Could you check a few things on this drawing? It's one solid part, dimensions in mm from its lowest x, y, z. A direction names the side the tool comes from. Give positions to 0.01 mm unless a question says otherwise; leave off trailing zeros. Order: outer loops, then holes, each group sorted by start corner. A loop starts at its lowest first (then second) coordinate and runs counter-clockwise, first axis right, second up.
(1) Imagine slicing it at D-D, the plane z = 2.5. Write out the boundary of the cut face in (x, y), then the cut area to 3 significant figures.
(2) If I drill on probe 1 along X at (y, z) = (46.85, 6); probe 2 along Z at (x, y) = (45, 48.2); probe 3 along Y at (x, z) = (14.5, 3), over which ranges is the centre line in solid material (lowest first)?
(3) On a 3-axis mill with a long thin cutter (end or side, diameter ignored), from which of +Z, -Z, +X, -X, +Y, -Y can I reach the whole of each face in a straight line? I mean the marked faces 5 and 6. Say none if no direction works.
(4) If we mould it in two halves opening along X, with no side actions, what happens to the marked faces 1, 2, 3 and 4? For each: released by +X, released by -X, zero draft, split by the parting line, or undercut.
(5) Imagine slicing it at A-A, the plane x = 25. Write out the boundary of the cut face in (y, z), then the cut area to 3 significant figures.
(6) Imagine slicing it at C-C, the plane x = 45. Write out the boundary of the cut face in (y, z).
(7) Will these pins go through, and if not, where does the flat tip stop? pin 1 (4 mm diameter, centred on x = 4, z = 6, fed in from +Y); pin 2 (1.5 mm diameter, centred on x = 45.5, z = 6.5, fed in from -Y).
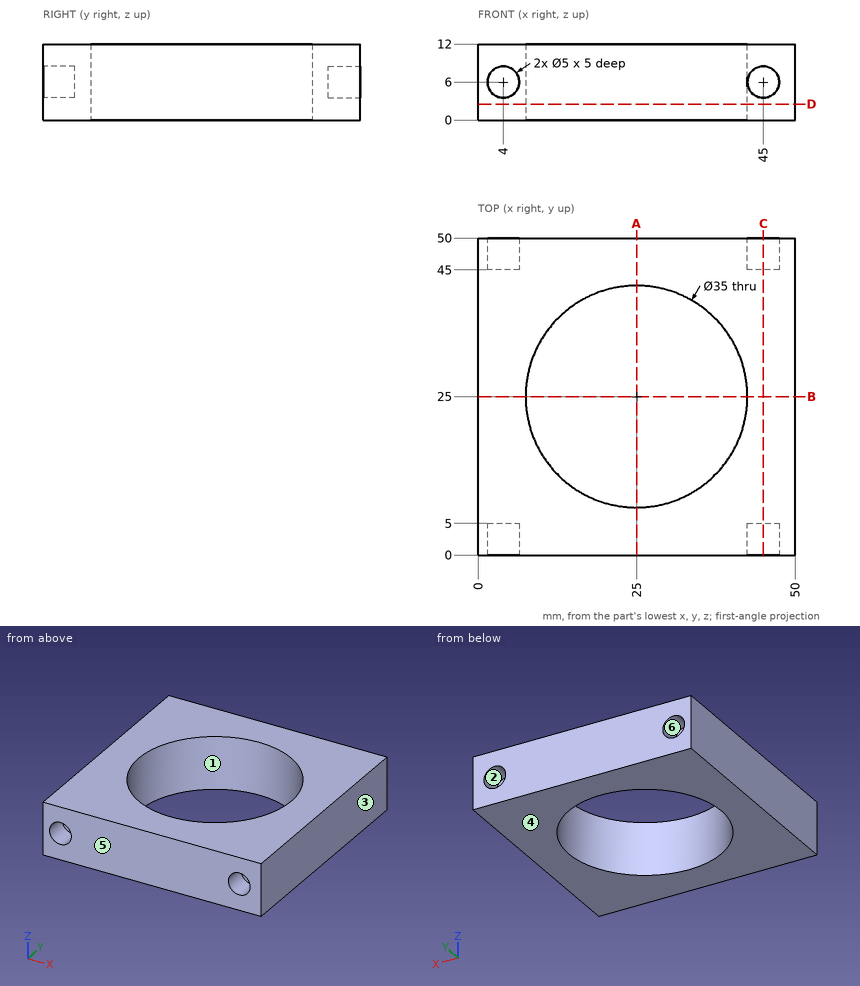
Answer block:
1. outline: (0, 0) - (50, 0) - (50, 50) - (0, 50) - close; hole circle Ø35 at (25, 25)
1. area: 1,540 mm2
2. probe 1: x = 0 to 1.5, 6.5 to 42.5, 47.5 to 50
2. probe 2: z = 0 to 3.5, 8.5 to 12
2. probe 3: y = 0 to 11, 39 to 50
3. face 5: +Z, -Z, +X, -X, -Y
3. face 6: +Y
4. face 1: undercut
4. face 2: undercut
4. face 3: released by +X
4. face 4: zero draft
5. outline: (0, 0) - (7.5, 0) - (7.5, 12) - (0, 12) - close; (42.5, 0) - (50, 0) - (50, 12) - (42.5, 12) - close
5. area: 180 mm2
6. outline: (0, 0) - (50, 0) - (50, 3.5) - (45, 3.5) - (45, 8.5) - (50, 8.5) - (50, 12) - (0, 12) - (0, 8.5) - (5, 8.5) - (5, 3.5) - (0, 3.5) - close
7. pin 1: stops at y = 45
7. pin 2: stops at y = 5
